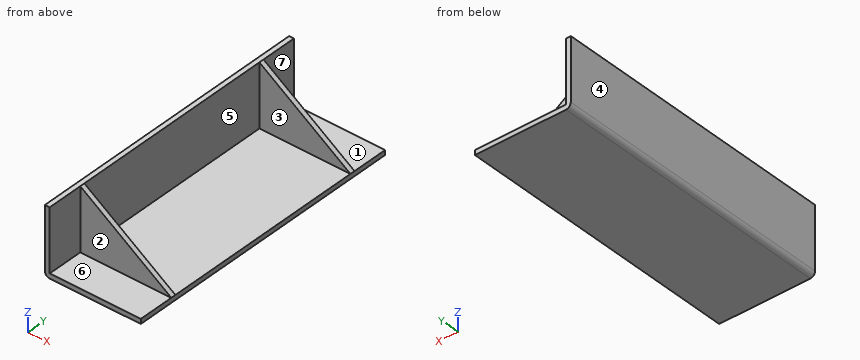
from build123d import *

# Parameters (mm, degrees)
SALIENTE_EXTRUIR1_DEPTH = 150
NERVIO1_REACH           = 289.228
CROQUIS2_WALL_W         = 691.564908986
CROQUIS2_WALL_H         = 5


with BuildPart() as part:
    # Croquis1 → Saliente-Extruir1 (new, symmetric)
    with BuildSketch(Plane(origin=(0, 0, 0), x_dir=(1, 0, 0), z_dir=(0, 1, 0))):
        with BuildLine():
            Line((5, 0), (100, 0))
            Line((100, 0), (100, -5))
            Line((100, -5), (5, -5))
            Line((5, -5), (5, -70))
            Line((5, -70), (0, -70))
            Line((0, -70), (0, -5))
            ThreePointArc((0, -5), (1.464466094, -1.464466094), (5, 0))
        make_face()
    extrude(amount=SALIENTE_EXTRUIR1_DEPTH, both=True)

    # Croquis2 wall → Nervio1 (add, up to next)
    with BuildSketch(Plane(origin=(52.5, 110, 37.5), x_dir=(-0.82530726125, 0, 0.564683915592), z_dir=(0.564683915592, 0, 0.82530726125)), mode=Mode.PRIVATE) as nervio1_sk1:
        Rectangle(CROQUIS2_WALL_W, CROQUIS2_WALL_H)
    nervio1_tool1 = extrude(nervio1_sk1.sketch, amount=-NERVIO1_REACH, mode=Mode.PRIVATE) - part.part
    nervio1 = nervio1_tool1.solids().sort_by_distance((52.5, 110, 37.5))[0]
    add(nervio1)

    # Simetría1: Nervio1 across plane
    add(nervio1.mirror(Plane.ZX))


solid = part.part
Part model, mm, in its own coordinate system. Face numbers are marked on the shaded views. A direction names the side the tool comes from. Give positions to 0.01 mm unless a question says otherwise; leave off trailing zeros. Loops run counter-clockwise (first coordinate to the right, second up) from the corner with the lowest first, then second, coordinate; pieces in that order, holes last. Notation, with made-up numbers: M 85.25,-38 L 139.25,-38 A27 cw 139.25,-21 Z; hole C 36,-18 d8. An arc over 180 degrees is marked long. Put each result on its own line as item: value. Start each with the question number.
1) 3-axis set-ups, long thin cutter, end or side, ignore diameter. For the marked faces 4, 5, 6 and 7: which of +Z, -Z, +X, -X, +Y, -Y reach the whole face in a straight line?
2) Flat gauge pins, fed straight in: pin 1 (2 mm diameter, centred on y = -20.5, z = 51.5, fed in from +X); pin 2 (1.5 mm diameter, centred on x = 39, y = -74.5, fed in from -Z); pin 3 (19.5 mm diameter, centred on x = 68.5, z = 43.5, fed in from +Y); pin 4 (1 mm diameter, centred on x = 26, y = 47, fed in from +Z). Where does each tip first touch, or does it go through?
3) Probe probe 1 along Y at (x, z) = (57, 26.5); probe 2 along Z at (x, y) = (27, 125.5). List the from-to ranges inside material, lowest first.
4) Saw through at C-C (x = 31). List the corners of the cut face in (y, z).
5) Saw through at B-B (z = 52). List the corners of the cut face in (x, y), then the cut area to 3 significant figures.
6) Saw through at A-A (y = -124.5). List the corners of the cut face in (x, z), then the cut area to 3 significant figures.
7) Pull direction Y, two halves, no side cores. Call the marked faces 1, 2 and 3: +Y half, -Y half, draft (parallel to the pull), parting line (faces both ways), or undercut.
Numbers:
1. face 4: +Z, -Z, -X, +Y, -Y
1. face 5: +Z, +X
1. face 6: +Z, +X, -Y
1. face 7: +Z, +X, +Y
2. pin 1: x = 5
2. pin 2: z = 0
2. pin 3: through
2. pin 4: z = 5
3. probe 1: -112.5 to -107.5, 107.5 to 112.5
3. probe 2: 0 to 5
4. outline: M -150,0 L 150,0 L 150,5 L 112.5,5 L 112.5,52.21 L 107.5,52.21 L 107.5,5 L -107.5,5 L -107.5,52.21 L -112.5,52.21 L -112.5,5 L -150,5 Z
5. outline: M 0,-150 L 5,-150 L 5,-112.5 L 31.31,-112.5 L 31.31,-107.5 L 5,-107.5 L 5,107.5 L 31.31,107.5 L 31.31,112.5 L 5,112.5 L 5,150 L 0,150 Z
5. area: 1,760 mm^2
6. outline: M 0,5 A5 ccw 5,0 L 100,0 L 100,5 L 5,5 L 5,70 L 0,70 Z
6. area: 820 mm^2
7. face 1: draft
7. face 2: -Y half
7. face 3: undercut
